Design review of the part built by this model. Coordinates are the model's own, in mm. Face numbers are marked on the shaded views. A direction names the side the tool comes from. Give positions to 0.01 mm unless a question says otherwise; leave off trailing zeros. Loops run counter-clockwise (first coordinate to the right, second up) from the corner with the lowest first, then second, coordinate; pieces in that order, holes last. Notation, with made-up numbers: M 80,28 L 88,28 A22 cw 88,44 Z; hole C 18.5,48 d3. An arc over 180 degrees is marked long. Use a Markdown table: item, result. Add a question column.
(1) Add section B-B, the plane x = 0. Give the boundary of the cut face in (y, z), then the cut area to 3 significant figures.
(2) Insertion check: pin 1 Ø5 at (x, z) = (14.5, 0) entering from -Y; pin 2 Ø6.5 at (x, z) = (0.5, -1.5) entering from +Y. Each pin has a flat end and moves straight along its axis. Give the tip position at first contact, or say it passes through.
(3) For probe 1 along Z at (x, y) = (0, -16.75); probe 2 along Z at (x, y) = (14.5, -12); probe 3 along X at (y, z) = (-2.25, -3.75), list the stretches that pass through material, from the lowest coordinate up.
(4) Draft analysis for pull direction X (two halves, no side actions). For the marked faces 3, 4 and 5, state which applies: pulls with the +X half, pulls with the -X half, needs draft (parallel to the pull), parting line crosses it, or undercut.
(5) Add section A-A, the plane y = -10. Give the boundary of the cut face in (x, z), then the cut area to 3 significant figures.
(6) Add section C-C, the plane z = 0. Give the boundary of the cut face in (x, y).
(7) Add section D-D, the plane z = -6.5. Give the boundary of the cut face in (x, y).
(8) For the marked faces 1 and 2, list the 3-axis set-ups (+Z, -Z, +X, -X, +Y, -Y) from which the entire face can be reached by the end or side of a thin tool; tool diameter is ignored.
```python
from build123d import *

# Parameters (mm, degrees)
SKETCH_W        = 50
SKETCH_H        = 20
PAD_DEPTH       = 20
SKETCH001_W     = 13
SKETCH001_H     = 15
POCKET_DEPTH    = 20.001
SKETCH002_R     = 4
SKETCH002_R_2   = 3
POCKET001_DEPTH = 5
POCKET002_DEPTH = 20.001


with BuildPart() as part:
    # Sketch → Pad (new body)
    with BuildSketch(Plane.XZ):
        Rectangle(SKETCH_W, SKETCH_H)
    extrude(amount=PAD_DEPTH)

    # Sketch001 (on Face1 of Pad) → Pocket (cut, through all)
    with BuildSketch(Plane(origin=(0, 0, 10), x_dir=(-1, 0, 0), z_dir=(0, 0, 1))):
        with Locations((0, 7.5)):
            Rectangle(SKETCH001_W, SKETCH001_H)
    extrude(amount=-POCKET_DEPTH, mode=Mode.SUBTRACT)

    # Sketch002 (on Face8 of Pocket) → Pocket001 (cut)
    with BuildSketch(Plane.XZ.offset(20)):
        Circle(SKETCH002_R)
        with Locations((-14.5, 0)):
            Circle(SKETCH002_R_2)
        with Locations((14.5, 0)):
            Circle(SKETCH002_R_2)
    extrude(amount=-POCKET001_DEPTH, mode=Mode.SUBTRACT)

    # Sketch002 (on Face8 of Pocket) → Pocket002 (cut, through all)
    with BuildSketch(Plane.XZ.offset(20)):
        Circle(SKETCH002_R)
        with Locations((-14.5, 0)):
            Circle(SKETCH002_R_2)
        with Locations((14.5, 0)):
            Circle(SKETCH002_R_2)
    extrude(amount=-POCKET002_DEPTH, mode=Mode.SUBTRACT)


solid = part.part
```
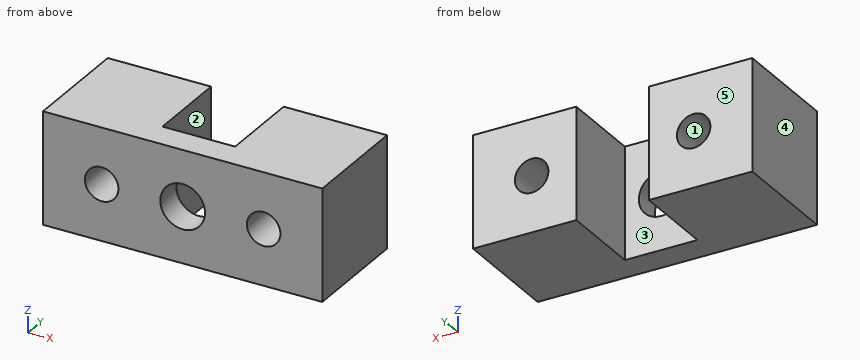
Established:
| question | item | result |
|---|---|---|
| 1 | outline | M -20,-10 L -15,-10 L -15,-4 L -20,-4 Z; M -20,4 L -15,4 L -15,10 L -20,10 Z |
| 1 | area | 60.0 mm^2 |
| 2 | pin 1 | through |
| 2 | pin 2 | y = -15 |
| 3 | probe 1 | -10 to -4, 4 to 10 |
| 3 | probe 2 | -10 to -3, 3 to 10 |
| 3 | probe 3 | -25 to -6.5, 6.5 to 25 |
| 4 | face 3 | undercut |
| 4 | face 4 | pulls with the -X half |
| 4 | face 5 | needs draft |
| 5 | outline | M -25,-10 L -6.5,-10 L -6.5,10 L -25,10 Z; M 6.5,-10 L 25,-10 L 25,10 L 6.5,10 Z; hole C -14.5,0 d6; hole C 14.5,0 d6 |
| 5 | area | 683 mm^2 |
| 6 | outline | M -25,-20 L -17.5,-20 L -17.5,0 L -25,0 Z; M -11.5,-20 L -4,-20 L -4,-15 L -6.5,-15 L -6.5,0 L -11.5,0 Z; M 4,-20 L 11.5,-20 L 11.5,0 L 6.5,0 L 6.5,-15 L 4,-15 Z; M 17.5,-20 L 25,-20 L 25,0 L 17.5,0 Z |
| 7 | outline | M -25,-20 L 25,-20 L 25,0 L 6.5,0 L 6.5,-15 L -6.5,-15 L -6.5,0 L -25,0 Z |
| 8 | face 1 | +Y, -Y |
| 8 | face 2 | +Z, -Z, +Y |
